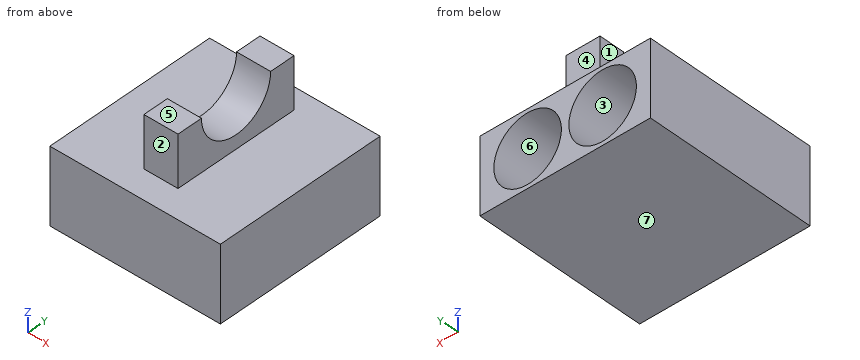
```python
from build123d import *

# Parameters (mm, degrees)
SKETCH1_W           = 50
SKETCH1_H           = 22
SKETCH1_R           = 9.89
BOSS_EXTRUDE1_DEPTH = 50.8
SKETCH2_R           = 10.5
BOSS_EXTRUDE2_DEPTH = 1
SKETCH3_R           = 10.5
BOSS_EXTRUDE3_DEPTH = 6.35
SKETCH5_W           = 10
SKETCH5_H           = 36.91
BOSS_EXTRUDE4_DEPTH = 15
SKETCH7_R           = 11
CUT_EXTRUDE1_DEPTH  = 10


with BuildPart() as part:
    # Sketch1 → Boss-Extrude1 (new body)
    with BuildSketch(Plane(origin=(0, 0, 0), x_dir=(1, 0, 0), z_dir=(0, 1, 0))):
        with Locations((4.998255194, -0.2362853)):
            Rectangle(SKETCH1_W, SKETCH1_H)
        with Locations((-6.001744806, -0.2362853)):
            Circle(SKETCH1_R, mode=Mode.SUBTRACT)
        with Locations((15.998255194, -0.2362853)):
            Circle(SKETCH1_R, mode=Mode.SUBTRACT)
    extrude(amount=BOSS_EXTRUDE1_DEPTH)

    # Sketch2 → Boss-Extrude2 (add)
    with BuildSketch(Plane(origin=(0, 0, 0), x_dir=(1, 0, 0), z_dir=(0, 1, 0))):
        with Locations((15.998255194, -0.2362853)):
            Circle(SKETCH2_R)
        with Locations((-6.001744806, -0.2362853)):
            Circle(SKETCH2_R)
    extrude(amount=BOSS_EXTRUDE2_DEPTH)

    # Sketch3 → Boss-Extrude3 (add)
    with BuildSketch(Plane(origin=(0, 1, 0), x_dir=(1, 0, 0), z_dir=(0, 1, 0))):
        with Locations((15.703735374, 0)):
            Circle(SKETCH3_R)
    extrude(amount=BOSS_EXTRUDE3_DEPTH)

    # Sketch5 → Boss-Extrude4 (add)
    with BuildSketch(Plane.XY.offset(11.2362853)):
        with Locations((5.231381217, 26.416579834)):
            Rectangle(SKETCH5_W, SKETCH5_H)
    extrude(amount=BOSS_EXTRUDE4_DEPTH)

    # Sketch7 → Cut-Extrude1 (cut)
    with BuildSketch(Plane(origin=(10.231381217, 0, 0), x_dir=(0, 0, -1), z_dir=(1, 0, 0))):
        with Locations((-26.2362853, 26.416579834)):
            Circle(SKETCH7_R)
    extrude(amount=-CUT_EXTRUDE1_DEPTH, mode=Mode.SUBTRACT)


solid = part.part
```
Could you check a few things on this model? Use its own coordinates, in mm. Face numbers are marked on the shaded views. A direction names the side the tool comes from. Round coordinates to 2 decimals unless told otherwise and drop trailing zeros. Loops run counter-clockwise (first coordinate to the right, second up) from the corner with the lowest first, then second, coordinate; pieces in that order, holes last. Notation, with made-up numbers: (62.5, 13.25) - (99.5, 13.25) arc R20 ccw to (99.5, 48.25) - close; hole circle Ø10 at (79, -0.75). An arc over 180 degrees is marked (long way). Answer in a Markdown table with one row per item. Add a question column.
(1) I need wall thicknesses on line 1 along X through (y, z) = (45.5, 2.5); line 2 along X through (y, z) = (27, 5); line 3 along X through (y, z) = (17, 12). Which ranges of each line are inside material? Lowest first, please.
(2) If we mould it in two halves opening along Z, with no side actions, what happens to the marked faces 4, 5, 6 and 7? For each: pulls with the +Z half, pulls with the -Z half, needs draft (parallel to the pull), parting line crosses it, or undercut.
(3) If we section it at A-A (z = 22.5): Please give me the cut outline in (x, y), plus the area to 3 significant figures.
(4) If we section it at B-B (y = 33.5): Please give me the cut outline in (x, z).
(5) If we section it at D-D (z = -3): Please give me the cut outline in (x, y), plus the area to 3 significant figures.
(6) I'm going to push flat-ended pins straight in: pin 1 (1 mm diameter, centred on y = 14.5, z = 16, fed in from -X); pin 2 (7.5 mm diameter, centred on y = 25.5, z = 22.5, fed in from +X); pin 3 (8 mm diameter, centred on x = 7.5, z = 19, fed in from -Y); pin 4 (18 mm diameter, centred on x = -6, z = 0.24, fed in from +Y). Where does each tip first touch, or does it pass through?
(7) For the marked faces 1, 2 and 3, which set-ups out of +Z, -Z, +X, -X, +Y, -Y let a thin tool reach every point of the face, with its end or its side?
(8) If we section it at C-C (x = 5): Please give me the cut outline in (y, z).
Model answer:
| question | item | result |
|---|---|---|
| 1 | line 1 | x = -20 to -15.63, 3.63 to 6.37, 25.63 to 30 |
| 1 | line 2 | x = -20 to -14.67, 2.67 to 7.33, 24.67 to 30 |
| 1 | line 3 | x = 0.23 to 10.23 |
| 2 | face 4 | needs draft |
| 2 | face 5 | pulls with the +Z half |
| 2 | face 6 | undercut |
| 2 | face 7 | pulls with the -Z half |
| 3 | outline | (0.23, 7.96) - (10.23, 7.96) - (10.23, 16.07) - (0.23, 16.07) - close; (0.23, 36.76) - (10.23, 36.76) - (10.23, 44.87) - (0.23, 44.87) - close |
| 3 | area | 162 mm² |
| 4 | outline | (-20, -10.76) - (30, -10.76) - (30, 11.24) - (10.23, 11.24) - (10.23, 17.82) - (0.23, 17.82) - (0.23, 11.24) - (-20, 11.24) - close; hole circle Ø19.78 at (-6, 0.24); hole circle Ø19.78 at (16, 0.24) |
| 5 | outline | (-20, 0) - (30, 0) - (30, 50.8) - (25.34, 50.8) - (25.34, 7.35) - (6.65, 7.35) - (6.65, 50.8) - (3.34, 50.8) - (3.34, 1) - (-15.35, 1) - (-15.35, 50.8) - (-20, 50.8) - close |
| 5 | area | 797 mm² |
| 6 | pin 1 | stops at x = 0.23 |
| 6 | pin 2 | passes through |
| 6 | pin 3 | stops at y = 7.96 |
| 6 | pin 4 | stops at y = 1 |
| 7 | face 1 | +Z, -X, +Y, -Y |
| 7 | face 2 | +Z, +X, -X, -Y |
| 7 | face 3 | +Y |
| 8 | outline | (0, -10.76) - (50.8, -10.76) - (50.8, 11.24) - (44.87, 11.24) - (44.87, 26.24) - (37.42, 26.24) arc R11 cw to (15.42, 26.24) - (7.96, 26.24) - (7.96, 11.24) - (0, 11.24) - close |
